```python
from build123d import *

# Parameters (mm, degrees)
SKIZZE1_R                            = 18
AUFSATZ_LINEAR_AUSTRAGEN1_DEPTH      = 5
SCHNITT_LINEAR_AUSTRAGEN1_DEPTH      = 26.942243542
SCHNITT_LINEAR_AUSTRAGEN1_DEPTH_BACK = 26.942243542
SKIZZE2_OUTSIDE_W                    = 48.232
SKIZZE2_OUTSIDE_H                    = 48.232
SKIZZE2_OUTSIDE_W_2                  = 36
SKIZZE2_OUTSIDE_H_2                  = 27.5
F_3_5_3_5_DURCHMESSER_BOHRUNG1_D     = 3.5
SCHNITT_LINEAR_AUSTRAGEN2_DEPTH      = 24.196174254
SCHNITT_LINEAR_AUSTRAGEN3_DEPTH      = 24.196174254
SKIZZE7_R                            = 3
SCHNITT_LINEAR_AUSTRAGEN4_DEPTH      = 22.5
F_1_5_1_5_DURCHMESSER_BOHRUNG1_D     = 1.5
VERRUNDUNG1_R                        = 0.6


with BuildPart() as part:
    # Skizze1 → Aufsatz-Linear austragen1 (new body)
    with BuildSketch(Plane(origin=(0, 0, 0), x_dir=(1, 0, 0), z_dir=(0, 1, 0))):
        with Locations(Location((0, 0, 0), (0, 0, 270))):
            Circle(SKIZZE1_R)
    extrude(amount=AUFSATZ_LINEAR_AUSTRAGEN1_DEPTH)

    # Skizze2 outside → Schnitt-Linear austragen1 (cut, two sides: drawn at the far end of the back side and taken through both)
    with BuildSketch(Plane(origin=(0, 5, 0), x_dir=(1, 0, 0), z_dir=(0, 1, 0)).offset(-SCHNITT_LINEAR_AUSTRAGEN1_DEPTH_BACK)):
        Rectangle(SKIZZE2_OUTSIDE_W, SKIZZE2_OUTSIDE_H)
        Rectangle(SKIZZE2_OUTSIDE_W_2, SKIZZE2_OUTSIDE_H_2, mode=Mode.SUBTRACT)
    extrude(amount=SCHNITT_LINEAR_AUSTRAGEN1_DEPTH + SCHNITT_LINEAR_AUSTRAGEN1_DEPTH_BACK, mode=Mode.SUBTRACT)

    # Ø3.5 (3.5) Durchmesser Bohrung1 (through all)
    with Locations(Plane(origin=(0, 5, 0), x_dir=(1, 0, 0), z_dir=(0, 1, 0))):
        with Locations((0, 10.9), (0, -10.9)):
            Hole(F_3_5_3_5_DURCHMESSER_BOHRUNG1_D / 2)

    # Skizze5 → Schnitt-Linear austragen2 (cut, through all)
    with BuildSketch(Plane(origin=(0, 5, 0), x_dir=(1, 0, 0), z_dir=(0, 1, 0))):
        with BuildLine():
            Line((-10.9, 7.65), (-17.888484908, 7.65))
            Line((-17.888484908, 7.65), (-17.888484908, 14.15))
            Line((-17.888484908, 14.15), (-7.65, 14.15))
            Line((-7.65, 14.15), (-7.65, 10.9))
            ThreePointArc((-7.65, 10.9), (-8.601902961, 8.601902961), (-10.9, 7.65))
        make_face()
        with BuildLine():
            Line((17.888484908, 14.15), (17.888484908, 7.65))
            Line((17.888484908, 7.65), (10.9, 7.65))
            ThreePointArc((10.9, 7.65), (8.601902961, 8.601902961), (7.65, 10.9))
            Line((7.65, 10.9), (7.65, 14.15))
            Line((7.65, 14.15), (17.888484908, 14.15))
        make_face()
        with BuildLine():
            Line((-17.888484908, -14.15), (-17.888484908, -7.65))
            Line((-17.888484908, -7.65), (-10.9, -7.65))
            ThreePointArc((-10.9, -7.65), (-8.601902961, -8.601902961), (-7.65, -10.9))
            Line((-7.65, -10.9), (-7.65, -14.15))
            Line((-7.65, -14.15), (-17.888484908, -14.15))
        make_face()
        with BuildLine():
            Line((10.9, -7.65), (17.888484908, -7.65))
            Line((17.888484908, -7.65), (17.888484908, -14.15))
            Line((17.888484908, -14.15), (7.65, -14.15))
            Line((7.65, -14.15), (7.65, -10.9))
            ThreePointArc((7.65, -10.9), (8.601902961, -8.601902961), (10.9, -7.65))
        make_face()
    extrude(amount=-SCHNITT_LINEAR_AUSTRAGEN2_DEPTH, mode=Mode.SUBTRACT)

    # Skizze6 → Schnitt-Linear austragen3 (cut, through all)
    with BuildSketch(Plane(origin=(0, 5, 0), x_dir=(1, 0, 0), z_dir=(0, 1, 0))):
        Polygon((6.350852961, 0), (3.175426481, 5.5), (-3.175426481, 5.5), (-6.350852961, 0), (-3.175426481, -5.5), (3.175426481, -5.5), align=None)
    extrude(amount=-SCHNITT_LINEAR_AUSTRAGEN3_DEPTH, mode=Mode.SUBTRACT)

    # Skizze7 → Schnitt-Linear austragen4 (cut, symmetric)
    with BuildSketch(Plane(origin=(0, 0, 0), x_dir=(0, 0, -1), z_dir=(1, 0, 0))):
        Circle(SKIZZE7_R)
    extrude(amount=SCHNITT_LINEAR_AUSTRAGEN4_DEPTH, both=True, mode=Mode.SUBTRACT)

    # Ø1.5 (1.5) Durchmesser Bohrung1 (through all)
    with Locations(Plane(origin=(0, 5, 0), x_dir=(1, 0, 0), z_dir=(0, 1, 0))):
        with Locations((3.175426481, 5.5), (-3.175426481, 5.5), (-6.350852961, 0), (-3.175426481, -5.5), (3.175426481, -5.5), (6.350852961, 0)):
            Hole(F_1_5_1_5_DURCHMESSER_BOHRUNG1_D / 2)

    # Verrundung1
    # the kernel refuses this fillet: 0.6 mm, written as the material it takes off along each edge
    with BuildSketch(Plane(origin=(-5.975852961, 6.148346656, -0.649519053), x_dir=(0.4999999999999993, 0, -0.8660254037844392), z_dir=(0, -1, 0))) as verrundung1_piece_1:
        with BuildLine():
            CenterArc((0.459338662, -0.6), VERRUNDUNG1_R, 90, 63.612200035)
            ThreePointArc((-0.078145188, -0.333333333), (-0.019797593, -0.171185412), (0, 0))
            Line((0, 0), (0.459338662, 0))
        make_face()
    extrude(amount=4.367849683, mode=Mode.SUBTRACT)
    with BuildSketch(Plane(origin=(-5.975852961, 6.148346656, 0.649519053), x_dir=(0.5000000000000006, 0, 0.8660254037844383), z_dir=(0, -1, 0)), Plane(origin=(5.975852961, 6.148346656, -0.649519053), x_dir=(-0.5000000000000003, 0, -0.8660254037844385), z_dir=(0, -1, 0))) as verrundung1_piece_2:
        with BuildLine():
            CenterArc((0.459338662, 0.6), VERRUNDUNG1_R, 206.387799965, 63.612200035)
            ThreePointArc((-0.078145188, 0.333333333), (-0.019797593, 0.171185412), (0, 0))
            Line((0, 0), (0.459338662, 0))
        make_face()
    extrude(amount=4.367849683, mode=Mode.SUBTRACT)
    with BuildSketch(Plane(origin=(-3.550426481, 6.148346656, 4.850480947), x_dir=(-0.49999999999999917, 0, -0.866025403784439), z_dir=(0, -1, 0)), Plane(origin=(3.550426481, 6.148346656, -4.850480947), x_dir=(0.5000000000000006, 0, 0.8660254037844383), z_dir=(0, -1, 0))) as verrundung1_piece_3:
        with BuildLine():
            CenterArc((0.459338662, -0.6), VERRUNDUNG1_R, 90, 63.612200058)
            ThreePointArc((-0.078145188, -0.333333334), (-0.019797593, -0.171185412), (0, 0))
            Line((0, 0), (0.459338662, 0))
        make_face()
    extrude(amount=7.296693312, mode=Mode.SUBTRACT)
    with BuildSketch(Plane(origin=(-2.425426481, 6.148346656, 5.5), x_dir=(-0.22824721632736633, 0, 0.9736032088272966), z_dir=(0, -1, 0)), Plane(origin=(2.425426481, 6.148346656, -5.5), x_dir=(0.22824721632736567, 0, -0.9736032088272967), z_dir=(0, -1, 0))) as verrundung1_piece_4:
        with BuildLine():
            CenterArc((0.479319154, -0.584161925), VERRUNDUNG1_R, 103.193899981, 63.612200039)
            Line((-0.104842771, -0.447213595), (0, 0))
            ThreePointArc((0, 0), (0.171185412, -0.019797593), (0.342370824, 0))
        make_face()
    extrude(amount=7.296693311, mode=Mode.SUBTRACT)
    with BuildSketch(Plane(origin=(2.425426481, 6.148346656, 5.5), x_dir=(-1, 0, 0), z_dir=(0, -1, 0)), Plane(origin=(-2.425426481, 6.148346656, -5.5), x_dir=(1, 0, 0), z_dir=(0, -1, 0))) as verrundung1_piece_5:
        with BuildLine():
            CenterArc((0.459338662, -0.6), VERRUNDUNG1_R, 90, 63.612200039)
            ThreePointArc((-0.078145188, -0.333333333), (-0.019797593, -0.171185412), (0, 0))
            Line((0, 0), (0.459338662, 0))
        make_face()
    extrude(amount=7.296693311, mode=Mode.SUBTRACT)
    with BuildSketch(Plane(origin=(3.550426481, 6.148346656, 4.850480947), x_dir=(0.7290415041794372, 0, 0.6844694917845379), z_dir=(0, -1, 0)), Plane(origin=(-3.550426481, 6.148346656, -4.850480947), x_dir=(-0.729041504179436, 0, -0.6844694917845393), z_dir=(0, -1, 0))) as verrundung1_piece_6:
        with BuildLine():
            CenterArc((0.479319154, -0.584161925), VERRUNDUNG1_R, 103.193899986, 63.612200058)
            Line((-0.104842771, -0.447213596), (0, 0))
            ThreePointArc((0, 0), (0.171185412, -0.019797593), (0.342370825, 0))
        make_face()
    extrude(amount=7.296693312, mode=Mode.SUBTRACT)
    with BuildSketch(Plane(origin=(5.975852961, 6.148346656, 0.649519053), x_dir=(0.9572887202373949, 0, 0.28913371665416454), z_dir=(0, -1, 0))) as verrundung1_piece_7:
        with BuildLine():
            CenterArc((0.479319154, 0.584161925), VERRUNDUNG1_R, 193.193899985, 63.612200035)
            Line((-0.104842771, 0.447213595), (0, 0))
            ThreePointArc((0, 0), (0.171185412, 0.019797593), (0.342370824, 0))
        make_face()
    extrude(amount=4.367849683, mode=Mode.SUBTRACT)


solid = part.part
```
The listing builds one solid part. Answer for the finished solid, in the listing's coordinates (mm). A direction names the side the tool comes from. Give positions to 0.01 mm unless a question says otherwise; leave off trailing zeros. Write each loop counter-clockwise with the first axis right and the second up, starting at its lowest first coordinate (ties: lowest second). Pieces come first, ordered by that corner, then holes. Notation, with made-up numbers: (11.5, 87.5) -> (59.5, 87.5) arc R8 cw to (59.5, 97.5) -> close; hole circle Ø8 at (50, 10.5). An arc over 180 degrees is marked (long way). Use one line per item in the form item = value.
1) Each of these flat-tipped pins is pushed along its axis until it touches: P1, Ø1.5, axis at x = -13, y = 3, coming from the -Z side; P2, Ø8, axis at x = 14, z = 2.5, coming from the -Y side; P3, Ø1.4, axis at y = 2.5, z = 12, coming from the +X side; P4, Ø2.5, axis at y = 3.5, z = 13, coming from the -X side. Where does it stop, or does it pass through?
Result:
P1 = -7.65
P2 = 0
P3 = 7.65
P4 = -7.65
2) Section C-C on y = 1.05 is taken. Count the separate pieces of the cut face and the enclosed holes in it, plus the area to 3 significant figures.
Result:
separate_pieces = 2
enclosed_holes = 2
area = 461 mm²
3) A tool of negligible diameter and unlimited length cuts with its end or side. For faces 1 (the flat face through (0, 3, 5.5)), 2 (the flat face through (-7.65, 3, 12)), 3 (the flat face through (14, 3, 7.65)), from which of +Z, -Z, +X, -X, +Y, -Y can it reach the whole face along a straight path? Write none if from no direction.
Result:
face_1 = +Y, -Y
face_2 = +Z, -X, +Y, -Y
face_3 = +Z, +X, +Y, -Y
4) Straight lines are drawn through the part: probe 1 along Z at (x, y) = (0, 2.65); probe 2 along X at (y, z) = (3.3, 10.9). For each, find the intervals that lie inside material, in ascending order.
Result:
probe_1 = -13.75 to -12.65, -9.15 to -5.5, 5.5 to 9.15, 12.65 to 13.75
probe_2 = -7.65 to -1.75, 1.75 to 7.65
5) For a pull along X with two mould halves and no side action, classify faces 4 (the cylindrical face through (-8.577, 2.535, -8.627)), 5 (the cylindrical face through (-3.535, 2.465, 6.158)), 6 (the flat face through (-4.53, 3.09, -3.15)), 7 (the flat face through (0, 5, 6)) as +X half, -X half, draft (parallel to the pull), parting line (faces both ways), or undercut.
Result:
face_4 = -X half
face_5 = undercut
face_6 = undercut
face_7 = draft
6) Section B-B on z = 0 is taken. Write down the section's boundary in (x, y).
Result:
outline = (-18, 3) -> (-7.1, 3) -> (-7.1, 5) -> (-18, 5) -> close; (7.1, 3) -> (18, 3) -> (18, 5) -> (7.1, 5) -> close
7) Section A-A on x = 0 is taken. Write down the section's boundary in (y, z).
Result:
outline = (0, -13.75) -> (5, -13.75) -> (5, -12.65) -> (0, -12.65) -> close; (0, -9.15) -> (5, -9.15) -> (5, -5.5) -> (0, -5.5) -> close; (0, 5.5) -> (5, 5.5) -> (5, 9.15) -> (0, 9.15) -> close; (0, 12.65) -> (5, 12.65) -> (5, 13.75) -> (0, 13.75) -> close
8) Section D-D on x = -5 is taken. Write down the section's boundary in (y, z).
Result:
outline = (0, -13.75) -> (5, -13.75) -> (5, -2.34) -> (1.88, -2.34) arc R3 cw to (0, -3) -> close; (0, 3) arc R3 cw to (1.88, 2.34) -> (5, 2.34) -> (5, 13.75) -> (0, 13.75) -> close
